For this review, take the finished solid that the model builds, in its own axes (mm). Give positions to 0.01 mm unless a question says otherwise; leave off trailing zeros. Loops run counter-clockwise (first coordinate to the right, second up) from the corner with the lowest first, then second, coordinate; pieces in that order, holes last. Notation, with made-up numbers: M 63.5,10.25 L 110.5,10.25 A12 ccw 110.5,21.25 Z; hole C 13,49.25 d4. An arc over 180 degrees is marked long. Use CSV: the item, a comma, the result in double quotes. Start each with the question number.
1. Take a section at B-B, the plane z = -16. Write out the cut boundary in (x, y).
2. To check wall thickness, follow line 1 (Y direction, x = -3, z = -26); line 2 (Y direction, x = 24, z = -7.5); line 3 (Z direction, x = 4, y = -18). State the ranges of each line that lie inside material, in increasing order. Write a range as [from, to].
3. Take a section at A-A, the plane x = 16.5. Write out the cut boundary in (y, z).
4. Insertion check: P1, Ø1.5, axis at x = 20.5, z = -2.5, coming from the -Y side; P2, Ø3, axis at x = -13, z = 26.5, coming from the +Y side; P3, Ø10.5, axis at x = 16, z = 16, coming from the +Y side. Each pin has a flat end and moves straight along its axis. Give the tip position at first contact, or say it passes through.
5. The part is to be moulded in two halves that separate along X. For faces 1 (the face through (0, -25, 0)), 2 (the face through (-0.59, -12.32, -4.46)), 3 (the face through (-13.581, 1.351, -12.206)), say which applies: pulls with the +X half, pulls with the -X half, needs draft (parallel to the pull), parting line crosses it, or undercut.
6. Take a section at C-C, the plane y = -20. Write out the cut boundary in (x, z).
7. Take a section at D-D, the plane z = -6.5. Write out the cut boundary in (x, y), and give its area (3 significant figures).
Autodesk Inventor part; units mm, degrees
ref_plane "YZ Plane" through (0, 0, 0) normal (1, 0, 0) x (0, 1, 0)
ref_plane "XZ Plane" through (0, 0, 0) normal (0, 1, 0) x (-1, 0, 0)
ref_plane "XY Plane" through (0, 0, 0) normal (0, 0, 1) x (1, 0, 0)
sketch "Sketch1" plane through (0, 0, 0) normal (0, 1, 0) x (-1, 0, 0)
  line L0 (37.5, -37.5) -> (-37.5, -37.5)
  line L1 (-37.5, -37.5) -> (-37.5, 37.5)
  line L2 (-37.5, 37.5) -> (37.5, 37.5)
  line L3 (37.5, 37.5) -> (37.5, -37.5)
  line L4 (37.5, -37.5) -> (-37.5, 37.5) construction
  line L5 (-37.5, -37.5) -> (37.5, 37.5) construction
  point P0 (0, 0)
  dimension "d0" = 75
  dimension "d1" = 75
sketch "Sketch2" plane through (0, 0, 0) normal (0, 1, 0) x (-1, 0, 0)
  line L0 (-25, -25) -> (25, -25)
  line L1 (25, -25) -> (25, 25)
  line L2 (25, 25) -> (-25, 25)
  line L3 (-25, 25) -> (-25, -25)
  line L4 (-25, -25) -> (25, 25) construction
  line L5 (25, -25) -> (-25, 25) construction
  point P0 (0, 0)
  dimension "d2" = 50
  dimension "d3" = 50
extrude "Extrusion1" add sketch "Sketch1" along normal blind 4
extrude "Extrusion2" [suppressed]
sketch "Sketch3" plane through (37.5, 0, 37.5) normal (1, 0, 0) x (0, 0, -1)
  line L0 (75, 4) -> (0, 4)
  line L1 (0, 0) -> (75, 0)
  line L2 (0, 0) -> (75, 0)
  arc A0 (75, 0) -> (0, 0) centre (37.5, -173.7812) ccw
  point P0 (37.5, 4)
extrude "Extrusion3" cut sketch "Sketch3" against normal through all keep common part
sketch "Sketch4" plane through (37.5, 0, -37.5) normal (0, 0, -1) x (-1, 0, 0)
  line L0 (75, 0) -> (75, 4)
  line L1 (0, 0) -> (75, 0)
  line L2 (0, 0) -> (0, 4)
  line L3 (75, 0) -> (0, 0)
  arc A0 (75, 0) -> (0, 0) centre (37.5, -173.7813) ccw
  point P0 (37.5, 0)
extrude "Extrusion4" cut sketch "Sketch4" against normal through all keep common part
sketch "Sketch5" plane through (0, 0, 0) normal (0, -1, 0) x (1, 0, 0)
  circle A0 centre (0, 0) radius 4.5
  dimension "d14" = 9
extrude "Extrusion5" add sketch "Sketch5" along normal blind 25
sketch "Sketch6" plane through (0, 0, 0) normal (0, -1, 0) x (1, 0, 0)
  circle A0 centre (-16, -16) radius 4.5
  circle A1 centre (16, 16) radius 4.5
  line L0 (0, 0) -> (37.5, 37.5)
  point P0 (0, 0)
  dimension "d17" = 9
  dimension "d18" = 9
  dimension "d19" = 16
  dimension "d20" = 16
  dimension "d21" = 16
  dimension "d22" = 16
extrude "Extrusion6" cut sketch "Sketch6" against normal through all
properties part number "thumper-bumper-trigger"
Result set:
1,outline,"M -37.5,0 L -20.5,0 L -20.5,2.81 A177.78 ccw Z; M -11.5,0 L 37.5,0 A177.78 ccw 16,3.28 L -11.5,3.28 Z"
2,line 1,"[0, 2.09]"
2,line 2,"[0, 2.37]"
2,line 3,"[-2.06, 2.06]"
3,outline,"M 0,-37.5 A177.78 ccw 3.23,-16.5 L 3.23,11.53 L 0,11.53 Z; M 0,20.47 L 2.82,20.47 A177.78 ccw 0,37.5 Z"
4,P1,"y = 0"
4,P2,"y = 2.23"
4,P3,"y = 3.57"
5,face 1,"needs draft"
5,face 2,"parting line crosses it"
5,face 3,"undercut"
6,outline,"C 0,0 d9"
7,outline,"M -37.5,0 L 37.5,0 A177.78 ccw 6.5,3.88 L -6.5,3.88 A177.78 ccw Z"
7,area,"199 mm2"
